Geometry: final body of the model. Coordinates: model frame, mm. Give positions to 0.01 mm unless a question says otherwise; leave off trailing zeros. Loops run counter-clockwise (first coordinate to the right, second up) from the corner with the lowest first, then second, coordinate; pieces in that order, holes last. Notation, with made-up numbers: (20, 73.5) -> (25, 73.5) arc R11 ccw to (25, 83.5) -> close; hole circle Ø5 at (44, 63.5). An arc over 180 degrees is marked (long way). Answer in a Markdown table with one row per item. Add a question column.
1) First-contact query: P1, Ø1.5, axis at x = 2, y = 117, coming from the +Z side; P2, Ø2, axis at x = 1, z = 6.5, coming from the +Y side; P3, Ø3, axis at x = -0.5, y = 26.5, coming from the -Z side. Flat tips, straight axial feed; report the tip coordinate or a pass-through.
2) Line query: line 1 (Z direction, x = 1.5, y = 158); line 2 (Y direction, x = 2.45, z = -2); line 3 (Y direction, x = -0.7, z = -7). Output: solid intervals per line, ascending. Write a range as from..to.
3) Section query C-C (z = 19.5). Return the cut outline in (x, y), plus the area to 3 significant figures.
4) Section query A-A (x = 1.8). Return the cut outline in (y, z).
5) Section query B-B (y = -157.5). Return the cut outline in (x, z), plus the area to 3 significant figures.
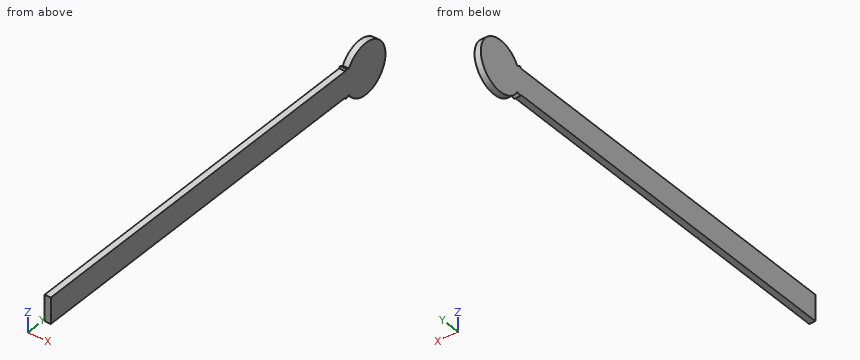
```python
from build123d import *

# Parameters (mm, degrees)
BOSS_EXTRUDE1_DEPTH = 3


with BuildPart() as part:
    # Sketch1 → Boss-Extrude1 (new body, symmetric)
    with BuildSketch(Plane(origin=(0, 0, 0), x_dir=(0, 0, -1), z_dir=(1, 0, 0))):
        with BuildLine():
            ThreePointArc((12.5, 175.728692494), (0, 221.3), (-12.5, 175.728692494))
            Line((-12.5, 175.728692494), (-12.5, 175.149364905))
            Line((-12.5, 175.149364905), (-14.25, 172.118275992))
            ThreePointArc((-14.25, 172.118275992), (-13.38309417, 171.637671204), (-12.5, 171.18750305))
            Line((-12.5, 171.18750305), (-12.5, -196.8))
            Line((-12.5, -196.8), (12.5, -196.8))
            Line((12.5, -196.8), (12.5, 171.18750305))
            ThreePointArc((12.5, 171.18750305), (13.38309417, 171.637671204), (14.25, 172.118275992))
            Line((14.25, 172.118275992), (12.5, 175.149364905))
            Line((12.5, 175.149364905), (12.5, 175.728692494))
        make_face()
    extrude(amount=BOSS_EXTRUDE1_DEPTH, both=True)


solid = part.part
```
Evaluation:
| question | item | result |
|---|---|---|
| 1 | P1 | z = 12.5 |
| 1 | P2 | y = 220.67 |
| 1 | P3 | z = -12.5 |
| 2 | line 1 | -12.5..12.5 |
| 2 | line 2 | -196.8..221.22 |
| 2 | line 3 | -196.8..220.28 |
| 3 | outline | (-3, 181.97) -> (3, 181.97) -> (3, 211.63) -> (-3, 211.63) -> close |
| 3 | area | 178 mm² |
| 4 | outline | (-196.8, -12.5) -> (171.19, -12.5) arc R28.5 ccw to (172.12, -14.25) -> (175.15, -12.5) -> (175.73, -12.5) arc R24.5 ccw (long way) to (175.73, 12.5) -> (175.15, 12.5) -> (172.12, 14.25) arc R28.5 ccw to (171.19, 12.5) -> (-196.8, 12.5) -> close |
| 5 | outline | (-3, -12.5) -> (3, -12.5) -> (3, 12.5) -> (-3, 12.5) -> close |
| 5 | area | 150 mm² |
